```python
from build123d import *

# Parameters (mm, degrees)
F0_W         = 30
F0_H         = 30
F1_DEPTH     = 5
F2_W         = 5
F2_H         = 15
F3_DEPTH     = 15
F4_R         = 2.4
F5_DEPTH     = 12
F6_R         = 2.5
F7_DEPTH     = 5
F8_SIZE      = 1
F9_R         = 5
F11_DEPTH    = 5
F12_T2_ANGLE = 359.64
F12_T4_ANGLE = 359.64
F13_DEPTH    = 7


# Not quite as in the source:
# - a fillet or chamfer that OpenCascade refuses, or shapes differently, is made with other operations: its cross-section is extruded or revolved along the edge and cut away or added


with BuildPart() as f1:
    # F0 (on Top) → F1 (new body)
    with BuildSketch(Plane.XY):
        with Locations((15, 15)):
            Rectangle(F0_W, F0_H)
    extrude(amount=F1_DEPTH)

    # F2 (on face) → F3 (join)
    with BuildSketch(Plane.XY.offset(5)):
        with Locations((17.5, 15)):
            Rectangle(F2_W, F2_H)
        with Locations((12.5, 15)):
            Rectangle(F2_W, F2_H)
    extrude(amount=F3_DEPTH)

    # F4 (on face) → F5 (join)
    with BuildSketch(Plane(origin=(10, 0, 0), x_dir=(0, -1, 0), z_dir=(-1, 0, 0))):
        with Locations((-15, 14)):
            Circle(F4_R)
    extrude(amount=F5_DEPTH)

    # F6 (on face) → F7 (cut, through all)
    with BuildSketch(Plane.XY.offset(5)):
        with Locations((25, 26.25)):
            Circle(F6_R)
        with Locations((5, 26.25)):
            Circle(F6_R)
        with Locations((5, 3.75)):
            Circle(F6_R)
        with Locations((25, 3.75)):
            Circle(F6_R)
    extrude(amount=-F7_DEPTH, mode=Mode.SUBTRACT)

    # F8
    f8_edges = [f1.edges().sort_by_distance(p)[0] for p in [
        (2.5, 26.25, 5),
        (22.5, 26.25, 5),
        (22.5, 3.75, 5),
        (2.5, 3.75, 5),
    ]]
    chamfer(f8_edges, length=F8_SIZE)

    # F9
    f9_edges = [f1.edges().sort_by_distance(p)[0] for p in [
        (15, 22.5, 20),
        (15, 7.5, 20),
    ]]
    fillet(f9_edges, radius=F9_R)

    # F10 (on face) → F11 (join)
    with BuildSketch(Plane(origin=(-2, 0, 0), x_dir=(0, -1, 0), z_dir=(-1, 0, 0))):
        with BuildLine():
            Line((-16, 16.1817424229), (-16, 17.3541019662))
            ThreePointArc((-16, 17.3541019662), (-18.5, 14), (-16, 10.6458980338))
            Line((-16, 10.6458980338), (-16, 11.8182575771))
            ThreePointArc((-16, 11.8182575771), (-17.4, 14), (-16, 16.1817424229))
        make_face()
        with BuildLine():
            ThreePointArc((-14, 10.6458980338), (-12.1937569599, 11.9083499337), (-11.5, 14))
            ThreePointArc((-11.5, 14), (-12.1937569599, 16.0916500663), (-14, 17.3541019662))
            Line((-14, 17.3541019662), (-14, 16.1817424229))
            ThreePointArc((-14, 16.1817424229), (-12.9800990123, 15.2961481397), (-12.6, 14))
            ThreePointArc((-12.6, 14), (-12.9800990123, 12.7038518603), (-14, 11.8182575771))
            Line((-14, 11.8182575771), (-14, 10.6458980338))
        make_face()
        with BuildLine():
            ThreePointArc((-12.6, 14), (-12.9800990123, 15.2961481397), (-14, 16.1817424229))
            Line((-14, 16.1817424229), (-14, 11.8182575771))
            ThreePointArc((-14, 11.8182575771), (-12.9800990123, 12.7038518603), (-12.6, 14))
        make_face()
        with BuildLine():
            Line((-16, 11.8182575771), (-16, 16.1817424229))
            ThreePointArc((-16, 16.1817424229), (-17.4, 14), (-16, 11.8182575771))
        make_face()
    extrude(amount=F11_DEPTH)

    # F12: fillet of radius 3 on 2 edges, made by hand

    # F12_s1 → F12_t2 (revolve, cut)
    with BuildSketch(Plane(origin=(0, 0.0441300513, 14.0469854057), x_dir=(1, 0, 0), z_dir=(0, -0.0031415875, -0.9999950652))):
        with BuildLine():
            ThreePointArc((-4, -11.4559437532), (-6.1213203436, -12.3346234097), (-7, -14.4559437532))
            Line((-7, -14.4559437532), (-7, -11.4559437532))
            Line((-7, -11.4559437532), (-4, -11.4559437532))
        make_face()
    revolve(axis=Axis((-7, 15, 14), (-1, 0, 0)), revolution_arc=F12_T2_ANGLE, mode=Mode.SUBTRACT)

    # F12_s3 → F12_t4 (revolve, cut)
    with BuildSketch(Plane(origin=(0, 0.0441300513, 14.0469854057), x_dir=(1, 0, 0), z_dir=(0, 0.0031415875, 0.9999950652))):
        with BuildLine():
            ThreePointArc((-4, 18.4559437532), (-6.1213203436, 17.5772640968), (-7, 15.4559437532))
            Line((-7, 15.4559437532), (-7, 18.4559437532))
            Line((-7, 18.4559437532), (-4, 18.4559437532))
        make_face()
    revolve(axis=Axis((-7, 15, 14), (-1, 0, 0)), revolution_arc=F12_T4_ANGLE, mode=Mode.SUBTRACT)

    # F13 (cut): a face of the model
    f13_faces = [f1.faces().sort_by_distance(p)[0] for p in [
        (-2, 15, 14),
    ]]
    extrude(f13_faces, amount=-F13_DEPTH, mode=Mode.SUBTRACT)


solid = f1.part
```
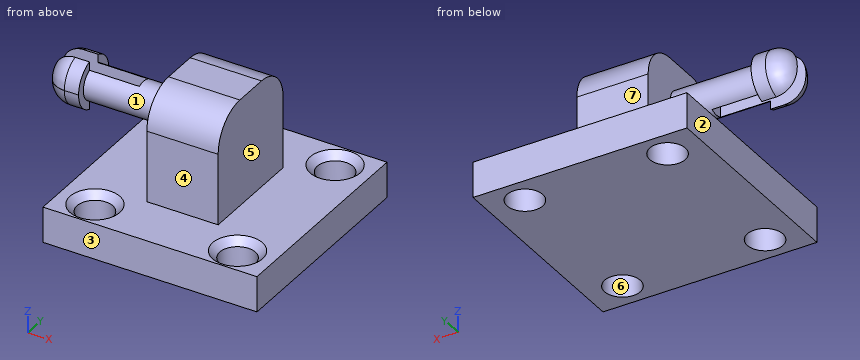
Source: CAD feature listing. Evaluate the final solid. Frame: model axes, mm. Face numbers are marked on the shaded views. A direction names the side the tool comes from. Give positions to 0.01 mm unless a question says otherwise; leave off trailing zeros. Order: outer loops, then holes, each group sorted by start corner. A loop starts at its lowest first (then second) coordinate and runs counter-clockwise, first axis right, second up.
(1) Section query D-D (z = 10). Return the cut outline in (x, y), plus the area to 3 significant figures.
(2) Section query A-A (y = 3.75). Return the cut outline in (x, z).
(3) Access query for the marked faces 4, 5, 6 and 7. Directions: +Z, -Z, +X, -X, +Y, -Y. A direction counts if a zero-diameter tool reaches every point of the face in a straight line with its end or side. Return the directions, or none.
(4) Section query C-C (y = 15). Return the cut outline in (x, z), plus the area to 3 significant figures.
(5) Section query B-B (x = 18). Return the cut outline in (y, z).
(6) Contact query for flat-ended pins moving along their axis: P1, Ø1.2, axis at y = 13.5, z = 13.5, coming from the +X side; P2, Ø2, axis at x = 17.5, y = 23, coming from the +Z side; P3, Ø4, axis at y = 16.5, z = 2, coming from the -X side. Output: stop coordinate, or through.
(7) Material intervals for line 1 along Y through (x, z) = (25, 1.1); line 2 along Z through (x, y) = (1, 24.5); line 3 along Y through (x, z) = (11, 10.25), sorted ascending.
(8) Pull-direction query (X, two-part tool) for the marked faces 1, 2 and 3; classes: +X half, -X half, draft (parallel to the pull), parting line (faces both ways), or undercut.
Outcome:
1. outline: (10, 7.5) - (20, 7.5) - (20, 22.5) - (10, 22.5) - close
1. area: 150 mm2
2. outline: (0, 0) - (2.5, 0) - (2.5, 4) - (1.5, 5) - (0, 5) - close; (7.5, 0) - (22.5, 0) - (22.5, 4) - (21.5, 5) - (8.5, 5) - (7.5, 4) - close; (27.5, 0) - (30, 0) - (30, 5) - (28.5, 5) - (27.5, 4) - close
3. face 4: +Z, +X, -X, -Y
3. face 5: +Z, +X, +Y, -Y
3. face 6: +Z, -Z
3. face 7: +Z, +X, -X, +Y
4. outline: (0, 0) - (30, 0) - (30, 5) - (20, 5) - (20, 20) - (10, 20) - (10, 16.4) - (5, 16.4) - (5, 11.6) - (10, 11.6) - (10, 5) - (0, 5) - close
4. area: 324 mm2
5. outline: (0, 0) - (30, 0) - (30, 5) - (22.5, 5) - (22.5, 15) arc R5 ccw to (17.5, 20) - (12.5, 20) arc R5 ccw to (7.5, 15) - (7.5, 5) - (0, 5) - close
6. P1: stops at x = 20
6. P2: stops at z = 17.18
6. P3: stops at x = 0
7. line 1: y = 0 to 1.25, 6.25 to 23.75, 28.75 to 30
7. line 2: z = 0 to 5
7. line 3: y = 7.5 to 22.5
8. face 1: undercut
8. face 2: -X half
8. face 3: draft
